from build123d import *

# Parameters (mm, degrees)
F0_W     = 122
F0_H     = 30
F1_DEPTH = 25
F2_R     = 7.5
F2_R_2   = 4.25
F3_DEPTH = 30
F4_W     = 62
F4_H     = 10
F5_DEPTH = 30
F6_R     = 1.5
F7_DEPTH = 7.5


with BuildPart() as f1:
    # F0 (on Top) → F1 (new body)
    with BuildSketch(Plane.XY):
        with Locations((6.373649, -27.108692)):
            Rectangle(F0_W, F0_H)
    extrude(amount=F1_DEPTH)

    # F2 (on face) → F3 (cut, through all)
    with BuildSketch(Plane.XZ.offset(42.108692)):
        with Locations((-37.126351, 14)):
            Circle(F2_R)
        with Locations((49.873649, 14)):
            Circle(F2_R)
        with Locations((6.373649, 14)):
            Circle(F2_R_2)
    extrude(amount=-F3_DEPTH, mode=Mode.SUBTRACT)

    # F4 (on face) → F5 (cut)
    with BuildSketch(Plane.XY.offset(25)):
        with Locations((6.373649, -17.108692)):
            Rectangle(F4_W, F4_H)
        with Locations((6.373649, -37.108692)):
            Rectangle(F4_W, F4_H)
    extrude(amount=-F5_DEPTH, mode=Mode.SUBTRACT)

    # F6 (on face) → F7 (cut)
    with BuildSketch(Plane.XY.offset(25)):
        with Locations((6.373649, -29.608692)):
            Circle(F6_R)
        with Locations((6.373649, -24.608692)):
            Circle(F6_R)
        with Locations((11.373649, -27.108692)):
            Circle(F6_R)
        with Locations((16.373649, -27.108692)):
            Circle(F6_R)
        with Locations((20.873649, -27.108692)):
            Circle(F6_R)
        with Locations((27.373649, -27.108692)):
            Circle(F6_R)
        with Locations((1.373649, -27.108692)):
            Circle(F6_R)
        with Locations((-3.626351, -27.108692)):
            Circle(F6_R)
        with Locations((-8.126351, -27.108692)):
            Circle(F6_R)
        with Locations((-14.626351, -27.108692)):
            Circle(F6_R)
    extrude(amount=-F7_DEPTH, mode=Mode.SUBTRACT)


solid = f1.part
Check sheet for the modelled part. Datum: model origin and axes. Units: mm. A direction names the side the tool comes from. Round coordinates to 2 decimals unless told otherwise and drop trailing zeros. Loops run counter-clockwise (first coordinate to the right, second up) from the corner with the lowest first, then second, coordinate; pieces in that order, holes last. Notation, with made-up numbers: M 26,61.25 L 47,61.25 A18 cw 47,66.25 Z; hole C -27.5,16 d2. An arc over 180 degrees is marked long. One line per question, with ' | ' between items. Start each with the question number.
Item 1: Scan lines: probe 1 along X at (y, z) = (-21, 23.25); probe 2 along Z at (x, y) = (-37, -24); probe 3 along X at (y, z) = (-20, 10). Record each from-to range of solid material in increasing order.
Item 2: Gauge pin test, flat ends, axial feed: pin 1 Ø1 at (x, z) = (-12, 7.5) entering from -Y; pin 2 Ø2.5 at (x, y) = (20.87, -27.11) entering from +Z; pin 3 Ø7.5 at (x, z) = (6.37, 14) entering from +Y; pin 4 Ø12 at (x, z) = (18.5, 21.5) entering from +Y. Record the tip position at first contact, or that the pin passes through.
Item 3: Section check A-A (y = -21). Record the boundary of the cut face in (x, z), and give its area (3 significant figures).
Item 4: Release check for a two-part mould opening along X. For faces 6 (the face through (-54.626, -27, 12)), 7 (the face through (11, -27, 17.5)), 8 (the face through (6, -27, 25)) record: released by +X, released by -X, zero draft, split by the parting line, or undercut.
Item 5: Set-up check for faces 1 (the face through (6, -27, 0)), 2 (the face through (6, -32.109, 7)), 3 (the face through (37.374, -17, 13)), 4 (the face through (21, -27, 17.5)), 5 (the face through (67.374, -27, 12)): record each of +Z, -Z, +X, -X, +Y, -Y from which the full face is reachable in a straight line by a thin tool's end or side.
Item 6: Section check B-B (z = 14). Record the boundary of the cut face in (x, y), and give its area (4 significant figures).
Worked out:
1) probe 1: -54.63 to -24.63, 37.37 to 67.37 | probe 2: 0 to 6.5, 21.5 to 25 | probe 3: -54.63 to -43.47, -30.78 to -24.63, 37.37 to 43.53, 56.22 to 67.37
2) pin 1: y = -32.11 | pin 2: z = 17.5 | pin 3: through | pin 4: y = -22.11
3) outline: M -54.63,0 L -24.63,0 L -24.63,25 L -54.63,25 Z; M 37.37,0 L 67.37,0 L 67.37,25 L 37.37,25 Z; hole C -37.13,14 d15; hole C 49.87,14 d15 | area: 1,150 mm^2
4) face 6: released by -X | face 7: undercut | face 8: zero draft
5) face 1: -Z, +X, -X, +Y, -Y | face 2: +Z, -Z, -Y | face 3: +Z, -Z, +Y | face 4: +Z | face 5: +Z, -Z, +X, +Y, -Y
6) outline: M -54.63,-42.11 L -44.63,-42.11 L -44.63,-12.11 L -54.63,-12.11 Z; M -29.63,-42.11 L -24.63,-42.11 L -24.63,-32.11 L 2.12,-32.11 L 2.12,-22.11 L -24.63,-22.11 L -24.63,-12.11 L -29.63,-12.11 Z; M 10.62,-32.11 L 37.37,-32.11 L 37.37,-42.11 L 42.37,-42.11 L 42.37,-12.11 L 37.37,-12.11 L 37.37,-22.11 L 10.62,-22.11 Z; M 57.37,-42.11 L 67.37,-42.11 L 67.37,-12.11 L 57.37,-12.11 Z | area: 1,435 mm^2
